from build123d import *

# Parameters (mm, degrees)
F0_R      = 21.2186083974
F1_DEPTH  = 152.4
F4_R      = 21.2186083974
F5_DEPTH  = 2540
F5_TAPER  = 10
F6_R      = 20.954815433
F7_DEPTH  = 120.98847
F9_R      = 21.2186083974
F10_DEPTH = 88.9
F10_TAPER = -10
F11_W     = 132.7950581908
F11_H     = 6.2676130328
F12_DEPTH = 182.63136


with BuildPart() as f1:
    # F0 (on Top) → F1 (new body)
    with BuildSketch(Plane.XY):
        Circle(F0_R)
    extrude(amount=F1_DEPTH)

    # F4 (on face) → F5 (join)
    with BuildSketch(Plane.XY.offset(152.4)):
        Circle(F4_R)
    extrude(amount=F5_DEPTH, taper=F5_TAPER)

    # F6 (on face) → F7 (join)
    with BuildSketch(Plane(origin=(0, 0, 0), x_dir=(1, 0, 0), z_dir=(0, 0, -1))):
        Circle(F6_R)
    extrude(amount=F7_DEPTH)

    # F9 (on face) → F10 (join)
    with BuildSketch(Plane(origin=(0, 0, -120.98847), x_dir=(1, 0, 0), z_dir=(0, 0, -1))):
        Circle(F9_R)
    extrude(amount=F10_DEPTH, taper=F10_TAPER)

    # F11 (on face) → F12 (join)
    with BuildSketch(Plane(origin=(0, 0, -209.88847), x_dir=(1, 0, 0), z_dir=(0, 0, -1))):
        with Locations((0.5875863135, 0.0979314791)):
            Rectangle(F11_W, F11_H)
    extrude(amount=-F12_DEPTH)


solid = f1.part
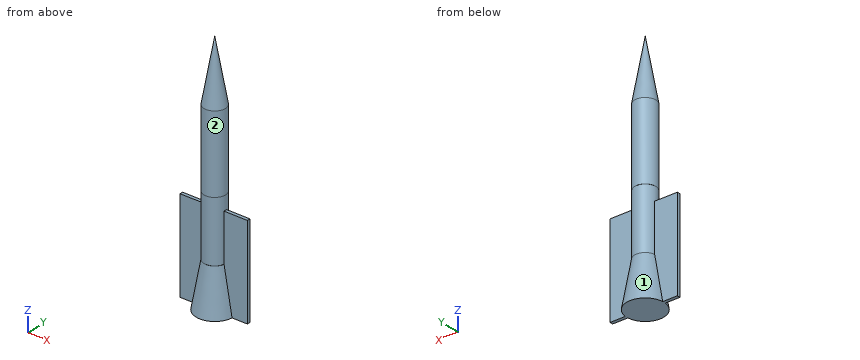
Can you work these out from the model? Positions are in its coordinate system, mm. Face numbers are marked on the shaded views. A direction names the side the tool comes from. Round coordinates to 2 decimals unless told otherwise and drop trailing zeros. Loops run counter-clockwise (first coordinate to the right, second up) from the corner with the lowest first, then second, coordinate; pieces in that order, holes last. Notation, with made-up numbers: (-36, -29) - (-16, -29) arc R21 cw to (-16, -21) - close; hole circle Ø10 at (71.25, -6). An arc over 180 degrees is marked (long way). Answer in a Markdown table with one row per item. Add a question column.
Q1. I want a section at A-A on z = -136. List the corners of the cut face in (x, y) for me, and give its area (3 significant figures).
Q2. Which directions (+Z, -Z, +X, -X, +Y, -Y) give clear straight access to the entire face, cutting with the end or side of a thin tool? Please do the marked faces 1 and 2.
Q3. For pin 1 Ø22.5 at (x, z) = (-42, -138.5) entering from -Y; pin 2 Ø6 at (y, z) = (22, 147.5) entering from +X; pin 3 Ø3 at (x, y) = (40, -1.5) entering from +Z; pin 4 Ø12 at (x, y) = (51, 12.5) entering from -Z, each with a flat end and sliding along its axis, tell me the tip position at first contact or that it passes through.
Q4. I want a section at C-C on z = 144.5. List the corners of the cut face in (x, y) for me.
Q5. I want a section at B-B on x = -53. List the corners of the cut face in (y, z) for me.
Q6. I need wall thicknesses on L1, parallel to Y at x = 38.5, z = -99.5; L2, parallel to X at y = -3.5, z = 54; L3, parallel to X at y = -4.5, z = 145.5. Which ranges of each line are inside material? Lowest first, please.
Q7. I want a section at D-D on z = 195. List the corners of the cut face in (x, y) for me.
A:
| question | item | result |
|---|---|---|
| 1 | outline | (-65.81, -3.23) - (-23.65, -3.23) arc R23.87 ccw to (23.65, -3.23) - (66.99, -3.23) - (66.99, 3.04) - (23.67, 3.04) arc R23.87 ccw to (-23.67, 3.04) - (-65.81, 3.04) - close |
| 1 | area | 2,320 mm^2 |
| 2 | face 1 | +Z, +Y |
| 2 | face 2 | +Z |
| 3 | pin 1 | y = -3.23 |
| 3 | pin 2 | x = 9.45 |
| 3 | pin 3 | z = -27.26 |
| 3 | pin 4 | through |
| 4 | outline | circle Ø42.44 at (0, 0) |
| 5 | outline | (-3.23, -209.89) - (3.04, -209.89) - (3.04, -27.26) - (-3.23, -27.26) - close |
| 6 | L1 | -3.23 to 3.04 |
| 6 | L2 | -20.93 to 20.93 |
| 6 | L3 | -20.74 to 20.74 |
| 7 | outline | circle Ø27.41 at (0, 0) |
